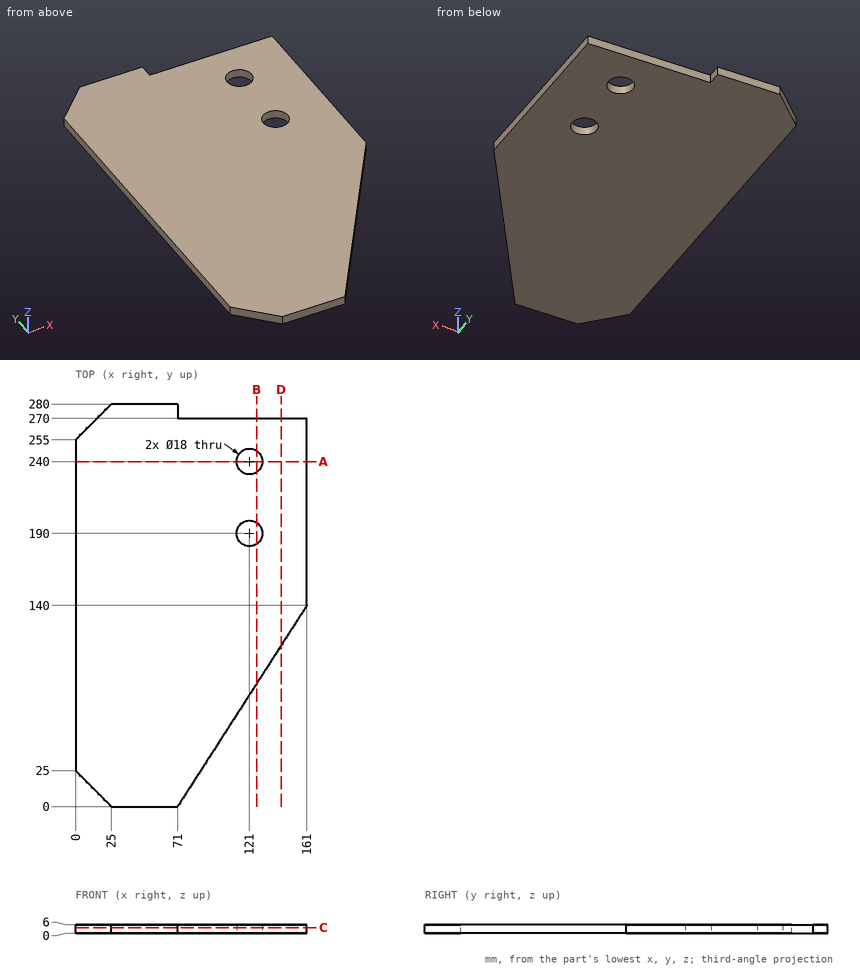
Can you work these out from the drawing? Everything is in mm from the part's minimum corner. Give positions to 0.01 mm unless a question says otherwise; leave off trailing zeros. Loops run counter-clockwise (first coordinate to the right, second up) from the corner with the lowest first, then second, coordinate; pieces in that order, holes last. Notation, with made-up numbers: (-29, -17) -> (-22, -17) arc R15 cw to (-22, -3) -> close; hole circle Ø3 at (-17, 41). An arc over 180 degrees is marked (long way). Write item = value, one per line.
1) Will these pins go through, and if not, where does the flat tip stop? pin 1 (11 mm diameter, centred on x = 121, y = 190, fed in from -Z); pin 2 (1 mm diameter, centred on y = 194, z = 1.5, fed in from -X); pin 3 (3 mm diameter, centred on y = 274.5, z = 2, fed in from +X); pin 4 (3 mm diameter, centred on x = 123.5, z = 4, fed in from +Y).
Check result:
pin_1 = through
pin_2 = 0
pin_3 = 71
pin_4 = 270
2) Suppose I cut it at B-B on x = 126. Write out the boundary of the cut face in (y, z), then the cut area to 3 significant figures.
Check result:
outline = (85.56, 0) -> (182.52, 0) -> (182.52, 6) -> (85.56, 6) -> close; (197.48, 0) -> (232.52, 0) -> (232.52, 6) -> (197.48, 6) -> close; (247.48, 0) -> (270, 0) -> (270, 6) -> (247.48, 6) -> close
area = 927 mm2
3) I need wall thicknesses on L1, parallel to X at y = 240, z = 2.6; L2, parallel to Y at x = 121, z = 4; L3, parallel to Y at x = 113, z = 3.5. Which ranges of each line are inside material? Lowest first, please. Write a range as from..to.
Check result:
L1 = 0..112, 130..161
L2 = 77.78..181, 199..231, 249..270
L3 = 65.33..185.88, 194.12..235.88, 244.12..270
4) Suppose I cut it at D-D on x = 143. Write out the boundary of the cut face in (y, z).
Check result:
outline = (112, 0) -> (270, 0) -> (270, 6) -> (112, 6) -> close
5) Suppose I cut it at C-C on z = 3.8. Write out the boundary of the cut face in (x, y), then the cut area to 3 significant figures.
Check result:
outline = (0, 25) -> (25, 0) -> (71, 0) -> (161, 140) -> (161, 270) -> (71, 270) -> (71, 280) -> (25, 280) -> (0, 255) -> close; hole circle Ø18 at (121, 190); hole circle Ø18 at (121, 240)
area = 36,700 mm2
6) Suppose I cut it at A-A on y = 240. Write out the boundary of the cut face in (x, z), then the cut area to 3 significant figures.
Check result:
outline = (0, 0) -> (112, 0) -> (112, 6) -> (0, 6) -> close; (130, 0) -> (161, 0) -> (161, 6) -> (130, 6) -> close
area = 858 mm2
